```python
from build123d import *

# Parameters (mm, degrees)
F0_W     = 150
F0_H     = 100
F0_R     = 8.064269
F1_DEPTH = 25


with BuildPart() as f1:
    # F0 (on Top) → F1 (new body)
    with BuildSketch(Plane.XY):
        with Locations((-0.348881, 7.363405)):
            Rectangle(F0_W, F0_H)
        with Locations((-61.726753, -32.127508)):
            Circle(F0_R, mode=Mode.SUBTRACT)
        with Locations((-41.726753, -32.127508)):
            Circle(F0_R, mode=Mode.SUBTRACT)
        with Locations((-21.726753, -32.127508)):
            Circle(F0_R, mode=Mode.SUBTRACT)
        with Locations((-1.726753, -32.127508)):
            Circle(F0_R, mode=Mode.SUBTRACT)
        with Locations((-61.726753, -7.127508)):
            Circle(F0_R, mode=Mode.SUBTRACT)
        with Locations((-41.726753, -7.127508)):
            Circle(F0_R, mode=Mode.SUBTRACT)
        with Locations((-21.726753, -7.127508)):
            Circle(F0_R, mode=Mode.SUBTRACT)
        with Locations((-1.726753, -7.127508)):
            Circle(F0_R, mode=Mode.SUBTRACT)
        with Locations((18.273247, -32.127508)):
            Circle(F0_R, mode=Mode.SUBTRACT)
        with Locations((38.273247, -32.127508)):
            Circle(F0_R, mode=Mode.SUBTRACT)
        with Locations((58.273247, -32.127508)):
            Circle(F0_R, mode=Mode.SUBTRACT)
        with Locations((18.273247, -7.127508)):
            Circle(F0_R, mode=Mode.SUBTRACT)
        with Locations((38.273247, -7.127508)):
            Circle(F0_R, mode=Mode.SUBTRACT)
        with Locations((58.273247, -7.127508)):
            Circle(F0_R, mode=Mode.SUBTRACT)
        with Locations((-61.726753, 17.872492)):
            Circle(F0_R, mode=Mode.SUBTRACT)
        with Locations((-41.726753, 17.872492)):
            Circle(F0_R, mode=Mode.SUBTRACT)
        with Locations((-21.726753, 17.872492)):
            Circle(F0_R, mode=Mode.SUBTRACT)
        with Locations((-1.726753, 17.872492)):
            Circle(F0_R, mode=Mode.SUBTRACT)
        with Locations((-61.726753, 42.872492)):
            Circle(F0_R, mode=Mode.SUBTRACT)
        with Locations((-41.726753, 42.872492)):
            Circle(F0_R, mode=Mode.SUBTRACT)
        with Locations((-21.726753, 42.872492)):
            Circle(F0_R, mode=Mode.SUBTRACT)
        with Locations((-1.726753, 42.872492)):
            Circle(F0_R, mode=Mode.SUBTRACT)
        with Locations((18.273247, 17.872492)):
            Circle(F0_R, mode=Mode.SUBTRACT)
        with Locations((38.273247, 17.872492)):
            Circle(F0_R, mode=Mode.SUBTRACT)
        with Locations((58.273247, 17.872492)):
            Circle(F0_R, mode=Mode.SUBTRACT)
        with Locations((18.273247, 42.872492)):
            Circle(F0_R, mode=Mode.SUBTRACT)
        with Locations((38.273247, 42.872492)):
            Circle(F0_R, mode=Mode.SUBTRACT)
        with Locations((58.273247, 42.872492)):
            Circle(F0_R, mode=Mode.SUBTRACT)
    extrude(amount=F1_DEPTH)


solid = f1.part
```
For this review, take the finished solid that the model builds, in its own axes (mm). Give positions to 0.01 mm unless a question says otherwise; leave off trailing zeros. Write each loop counter-clockwise with the first axis right and the second up, starting at its lowest first coordinate (ties: lowest second). Pieces come first, ordered by that corner, then holes.
Item 1: Insertion check: P1, Ø18.5, axis at x = -61.73, y = 42.87, coming from the +Z side. The pin has a flat end and moves straight along its axis. Give the tip position at first contact, or say it passes through.
Item 2: Wall thickness on probe 1 along Y at (x, z) = (-61, 22.5); probe 2 along Y at (x, z) = (40.5, 17.25): over which ranges is each line inside the solid? List them lowest first.
Item 3: Take a section at A-A (x = 14). Give the boundary of the cut face in (y, z), and give its area (3 significant figures).
Item 4: The part is to be moulded in two halves that separate along X. For faces 1 (the face through (-75.349, 7, 12)), 2 (the face through (74.651, 7, 12)), 3 (the face through (50.217, 43.227, 12.325)), say which applies: +X half, -X half, draft (parallel to the pull), parting line (faces both ways), or undercut.
Item 5: Take a section at D-D (x = -57). Give the boundary of the cut face in (y, z).
Item 6: Take a section at B-B (y = 14.5). Give the number of separate pieces and of enclosed holes in the cut face, and give its area (3 significant figures).
Established:
1. P1: stops at z = 25
2. probe 1: y = -42.64 to -40.16, -24.1 to -15.16, 0.9 to 9.84, 25.9 to 34.84, 50.9 to 57.36
2. probe 2: y = -42.64 to -39.88, -24.38 to -14.88, 0.62 to 10.12, 25.62 to 35.12, 50.62 to 57.36
3. outline: (-42.64, 0) - (-38.97, 0) - (-38.97, 25) - (-42.64, 25) - close; (-25.29, 0) - (-13.97, 0) - (-13.97, 25) - (-25.29, 25) - close; (-0.29, 0) - (11.03, 0) - (11.03, 25) - (-0.29, 25) - close; (24.71, 0) - (36.03, 0) - (36.03, 25) - (24.71, 25) - close; (49.71, 0) - (57.36, 0) - (57.36, 25) - (49.71, 25) - close
3. area: 1,130 mm2
4. face 1: -X half
4. face 2: +X half
4. face 3: undercut
5. outline: (-42.64, 0) - (-38.66, 0) - (-38.66, 25) - (-42.64, 25) - close; (-25.59, 0) - (-13.66, 0) - (-13.66, 25) - (-25.59, 25) - close; (-0.59, 0) - (11.34, 0) - (11.34, 25) - (-0.59, 25) - close; (24.41, 0) - (36.34, 0) - (36.34, 25) - (24.41, 25) - close; (49.41, 0) - (57.36, 0) - (57.36, 25) - (49.41, 25) - close
6. separate pieces: 8
6. enclosed holes: 0
6. area: 1,190 mm2
